Work out the finished part from the listing and answer in its coordinate system (mm). Face numbers are marked on the shaded views. A direction names the side the tool comes from. Round coordinates to 2 decimals unless told otherwise and drop trailing zeros. Loops run counter-clockwise (first coordinate to the right, second up) from the corner with the lowest first, then second, coordinate; pieces in that order, holes last. Notation, with made-up numbers: (70.5, -18.5) - (106.5, -18.5) arc R15 cw to (106.5, -14.5) - close; hole circle Ø2 at (85, 78). An arc over 180 degrees is marked (long way). Answer as CSV lines item,"result". Start each with the question number.
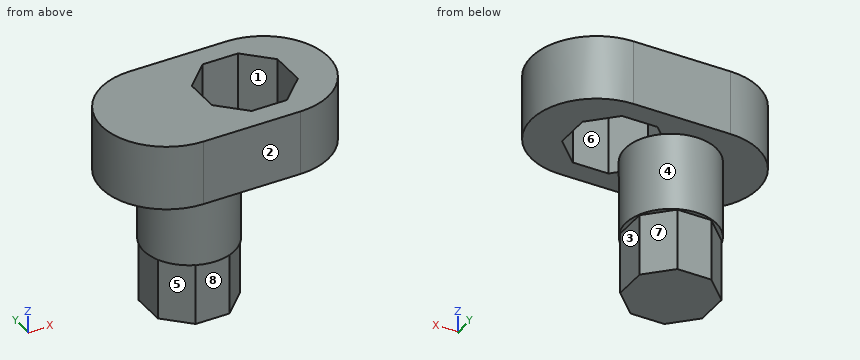
```python
from build123d import *

# Parameters (mm, degrees)
PAD_DEPTH    = 40
POCKET_DEPTH = 100
SKETCH002_R  = 28
PAD001_DEPTH = 48
PAD002_DEPTH = 38


with BuildPart() as part:
    # Sketch → Pad (new body)
    with BuildSketch(Plane.XY):
        with BuildLine():
            Line((-30, 40), (30, 40))
            ThreePointArc((30, -40), (70, 0), (30, 40))
            Line((-30, -40), (30, -40))
            ThreePointArc((-30, 40), (-70, 0), (-30, -40))
        make_face()
    extrude(amount=PAD_DEPTH)

    # Sketch001 (on DatumPlane) → Pocket (cut)
    with BuildSketch(Plane(origin=(0, 0, 0), x_dir=(1, 0, 0), z_dir=(0, 0, -1))):
        Polygon((29.443651, -26.556349), (45, -11), (45, 11), (29.443651, 26.556349), (7.443651, 26.556349), (-8.112698, 11), (-8.112698, -11), (7.443651, -26.556349), align=None)
    extrude(amount=-POCKET_DEPTH, mode=Mode.SUBTRACT)

    # Sketch002 (on DatumPlane) → Pad001 (join)
    with BuildSketch(Plane(origin=(0, 0, 0), x_dir=(1, 0, 0), z_dir=(0, 0, -1))):
        with Locations((-16, 0)):
            Circle(SKETCH002_R)
    extrude(amount=PAD001_DEPTH)

    # Sketch003 (on DatumPlane) → Pad002 (join)
    with BuildSketch(Plane(origin=(0, 0, -48), x_dir=(1, 0, 0), z_dir=(0, 0, -1))):
        Polygon((-5.5, -25.349242), (9.349242, -10.5), (9.349242, 10.5), (-5.5, 25.349242), (-26.5, 25.349242), (-41.349242, 10.5), (-41.349242, -10.5), (-26.5, -25.349242), align=None)
    extrude(amount=PAD002_DEPTH)


solid = part.part
```
Item 1: Which of the six approach directions +Z, -Z, +X, -X, +Y, -Y give full straight-line access (tool end or side, diameter ignored) to the marked faces 5, 6, 7 and 8?
Item 2: Flat-ended cylindrical pins translate along their axes: pin 1 Ø8 at (y, z) = (-28, -40.5) entering from +X; pin 2 Ø6 at (x, y) = (2, 8.5) entering from +Z; pin 3 Ø5 at (y, z) = (0.5, -61) entering from +X. Find the tip coordinate at first contact, or state that the pin passes through.
Item 3: Section D-D, the plane z = -63 is taken. Give the vertices of the cut face in (x, y).
Item 4: Section A-A, the plane z = 27 is taken. Give the vertices of the cut face in (x, y), and give its area (3 significant figures).
Item 5: Find the intervals of material crossed by L1, parallel to Z at x = -38.5, y = -24; L2, parallel to X at y = 6, z = -64; L3, parallel to Y at x = 5, z = 11.5, in increasing order.
Item 6: Section C-C, the plane x = 15 is taken. Give the vertices of the cut face in (y, z), and give its area (3 significant figures).
Item 7: Determine the mould class of the marked faces 1, 2, 3 and 4 for opening direction X: pulls with the +X half, pulls with the -X half, needs draft (parallel to the pull), parting line crosses it, or undercut.
Item 8: Section B-B, the plane y = 0 is taken. Give the vertices of the cut face in (x, z).
Answer:
1,face 5,"-Z, -X, -Y"
1,face 6,"+Z, -Z"
1,face 7,"-Z, +X, +Y"
1,face 8,"-Z, +X, -X, -Y"
2,pin 1,"stops at x = -1.58"
2,pin 2,"stops at z = 0"
2,pin 3,"stops at x = 9.35"
3,outline,"(-41.35, -10.5) - (-26.5, -25.35) - (-5.5, -25.35) - (9.35, -10.5) - (9.35, 10.5) - (-5.5, 25.35) - (-26.5, 25.35) - (-41.35, 10.5) - close"
4,outline,"(-30, -40) - (30, -40) arc R40 ccw to (30, 40) - (-30, 40) arc R40 ccw to start; hole (-8.11, -11) - (7.44, -26.56) - (29.44, -26.56) - (45, -11) - (45, 11) - (29.44, 26.56) - (7.44, 26.56) - (-8.11, 11) - close"
4,area,"7,490 mm²"
5,L1,"z = 0 to 40"
5,L2,"x = -41.35 to 9.35"
5,L3,"y = -40 to -24.11, 24.11 to 40"
6,outline,"(-40, 0) - (-26.56, 0) - (-26.56, 40) - (-40, 40) - close; (26.56, 0) - (40, 0) - (40, 40) - (26.56, 40) - close"
6,area,"1,080 mm²"
7,face 1,"undercut"
7,face 2,"needs draft"
7,face 3,"pulls with the +X half"
7,face 4,"parting line crosses it"
8,outline,"(-70, 0) - (-44, 0) - (-44, -48) - (-41.35, -48) - (-41.35, -86) - (9.35, -86) - (9.35, -48) - (12, -48) - (12, 0) - (-8.11, 0) - (-8.11, 40) - (-70, 40) - close; (45, 0) - (70, 0) - (70, 40) - (45, 40) - close"
